For this review, take the finished solid that the model builds, in its own axes (mm). A direction names the side the tool comes from. Give positions to 0.01 mm unless a question says otherwise; leave off trailing zeros. Write each loop counter-clockwise with the first axis right and the second up, starting at its lowest first coordinate (ties: lowest second). Pieces come first, ordered by that corner, then holes. Notation, with made-up numbers: (-7.5, 66) -> (11.5, 66) arc R20 ccw to (11.5, 80) -> close; hole circle Ø7 at (23, 87.5). An arc over 180 degrees is marked (long way). Write item = value, one per line.
```python
from build123d import *

# Parameters (mm, degrees)
F1_DEPTH = 22.225
F2_R     = 5.08
F3_R     = 6.35
F4_R     = 7.14375
F5_DEPTH = 152.401
F6_R     = 7.14375
F7_DEPTH = 76.301927


with BuildPart() as f1:
    # F0 (on Front) → F1 (new body, symmetric)
    with BuildSketch(Plane.XZ):
        Polygon((-76.300927, 152.4), (-76.300927, 0), (-69.950927, 0), (-69.950927, 146.05), (291.999073, 146.05), (291.999073, 152.4), align=None)
    extrude(amount=F1_DEPTH, both=True)

    # F2
    f2_edges = [f1.edges().sort_by_distance(p)[0] for p in [
        (-69.950927, 0, 146.05),
    ]]
    fillet(f2_edges, radius=F2_R)

    # F3
    f3_edges = [f1.edges().sort_by_distance(p)[0] for p in [
        (-76.300927, 0, 152.4),
    ]]
    fillet(f3_edges, radius=F3_R)

    # F4 (on Top) → F5 (cut, through all)
    with BuildSketch(Plane.XY):
        with Locations((261.836573, 0)):
            Circle(F4_R)
        with Locations((-46.138427, 0)):
            Circle(F4_R)
    extrude(amount=F5_DEPTH, mode=Mode.SUBTRACT)

    # F6 (on Right) → F7 (cut, through all)
    with BuildSketch(Plane.YZ):
        with Locations((0, 125.4125)):
            Circle(F6_R)
        with Locations((0, 61.9125)):
            Circle(F6_R)
    extrude(amount=-F7_DEPTH, mode=Mode.SUBTRACT)


solid = f1.part
```
(1) Tool access review of faces 1 (the face through (268.436, -2.736, 149.181)), 2 (the face through (-69.951, -0.3, 69.5)): name each direction out of +Z, -Z, +X, -X, +Y, -Y from which nothing blocks a thin tool from reaching the whole face with its end or side.
Answers below:
face_1 = +Z, -Z
face_2 = -Z, +X, +Y, -Y
(2) The part is to be moulded in two halves that separate along Y. For faces 3 (the face through (25, 22.225, 150)), 4 (the face through (-73.1, -0.9, 132.5)), 5 (the face through (-76.301, 0, 74)), 6 (the face through (25, -22.225, 150)), say which applies: released by +Y, released by -Y, zero draft, split by the parting line, or undercut.
Answers below:
face_3 = released by +Y
face_4 = undercut
face_5 = zero draft
face_6 = released by -Y
(3) For pin 1 (12 mm diameter, centred on x = 168, y = 12.5, fed in from -Z); pin 2 (11.5 mm diameter, centred on y = 0, z = 125.41, fed in from +X); pin 3 (22 mm diameter, centred on y = -6, z = 93.5, fed in from +X), all flat-tipped, find the tip position at first contact; note any pin that passes through.
Answers below:
pin_1 = 146.05
pin_2 = through
pin_3 = -69.95
(4) Take a section at B-B (x = -42.5). Write out the cut boundary in (y, z) (3 decimals).
Answers below:
outline = (-22.225, 146.05) -> (-6.148, 146.05) -> (-6.148, 152.4) -> (-22.225, 152.4) -> close; (6.148, 146.05) -> (22.225, 146.05) -> (22.225, 152.4) -> (6.148, 152.4) -> close
(5) Take a section at A-A (y = 0). Write out the cut boundary in (x, z).
Answers below:
outline = (-76.3, 0) -> (-69.95, 0) -> (-69.95, 54.77) -> (-76.3, 54.77) -> close; (-76.3, 69.06) -> (-69.95, 69.06) -> (-69.95, 118.27) -> (-76.3, 118.27) -> close; (-76.3, 132.56) -> (-69.95, 132.56) -> (-69.95, 140.97) arc R5.08 cw to (-64.87, 146.05) -> (-53.28, 146.05) -> (-53.28, 152.4) -> (-69.95, 152.4) arc R6.35 ccw to (-76.3, 146.05) -> close; (-38.99, 146.05) -> (254.69, 146.05) -> (254.69, 152.4) -> (-38.99, 152.4) -> close; (268.98, 146.05) -> (292, 146.05) -> (292, 152.4) -> (268.98, 152.4) -> close
(6) To check wall thickness, follow probe 1 along X at (y, z) = (0, 148.5); probe 2 along Z at (x, y) = (-71.25, 0); probe 3 along X at (y, z) = (4, 15). State the ranges of each line that lie inside material, in increasing order.
Answers below:
probe_1 = -75.81 to -53.28, -38.99 to 254.69, 268.98 to 292
probe_2 = 0 to 54.77, 69.06 to 118.27, 132.56 to 152.27
probe_3 = -76.3 to -69.95
(7) Take a section at C-C (z = 38.5). Write out the cut boundary in (x, y) (3 decimals), plus the area to 3 significant figures.
Answers below:
outline = (-76.301, -22.225) -> (-69.951, -22.225) -> (-69.951, 22.225) -> (-76.301, 22.225) -> close
area = 282 mm^2
